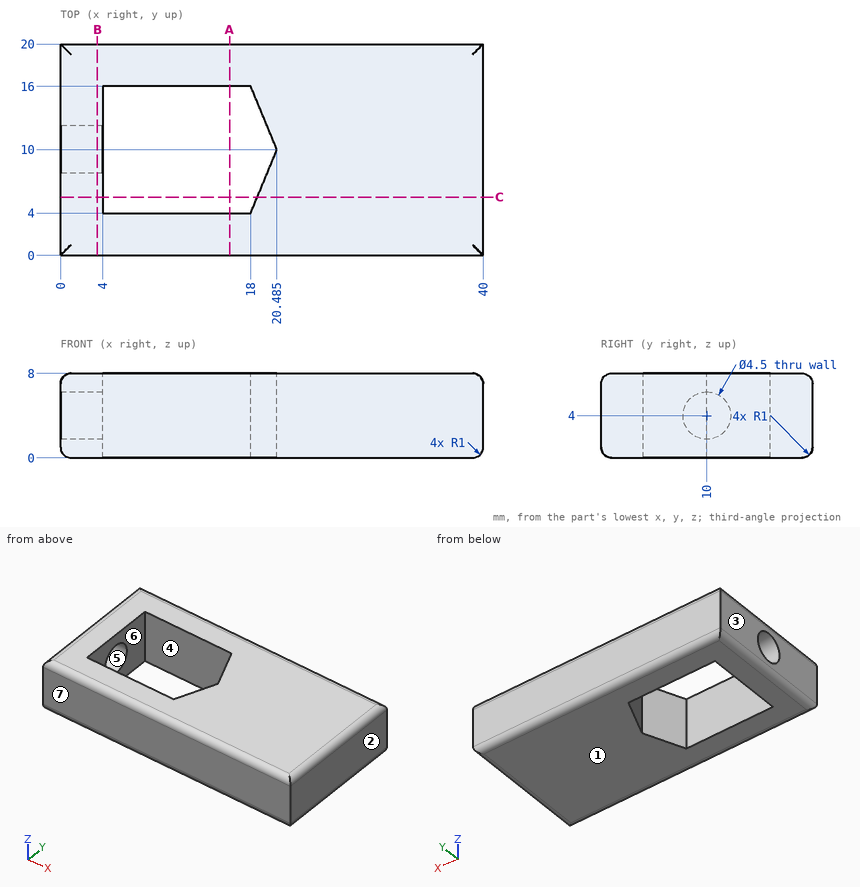
Study the drawing (mm; zero at the part's minimum x, y, z) and answer. A direction names the side the tool comes from. Coordinates: 2 decimals unless noted, no trailing zeros. Order: outer loops, then holes, each group sorted by start corner. A loop starts at its lowest first (then second) coordinate and runs counter-clockwise, first axis right, second up. Notation, with made-up numbers: M 68.5,66 L 127.5,66 A17 cw 127.5,81 Z; hole C -23,-14.5 d3. An arc over 180 degrees is marked long. Answer as a JSON object with one key per item and string values. Group by question number.
1. Section A-A on x = 16 is taken. Write down the section's boundary in (y, z).
2. Determine the mould class of the marked faces 1, 2, 3 and 4 for opening direction X: released by +X, released by -X, zero draft, split by the parting line, or undercut.
3. Straight lines are drawn through the part: line 1 (Y direction, x = 1.95, z = 4); line 2 (Y direction, x = 6.5, z = 1); line 3 (X direction, y = 4.25, z = 1.5). For each, find the intervals that lie inside material, in ascending order.
4. A flat-ended cylindrical pin translates along its axis: P1, Ø12, axis at x = 20, y = 9, coming from the +Z side. Find the tip coordinate at first contact, or state that the pin passes through.
5. A tool of negligible diameter and unlimited length cuts with its end or side. For the marked faces 5, 6 and 7, from which of +Z, -Z, +X, -X, +Y, -Y can it reach the whole face along a straight path? Write none if from no direction.
6. Section C-C on y = 5.5 is taken. Write down the section's boundary in (x, z), then the cut area to 3 significant figures.
7. Section B-B on x = 3.5 is taken. Write down the section's boundary in (y, z), then the cut area to 3 significant figures.
Values follow:
{
 "1": {"outline": "M 0,1 A1 ccw 1,0 L 4,0 L 4,8 L 1,8 A1 ccw 0,7 Z; M 16,0 L 19,0 A1 ccw 20,1 L 20,7 A1 ccw 19,8 L 16,8 Z"},
 "2": {"face 1": "zero draft", "face 2": "released by +X", "face 3": "released by -X", "face 4": "undercut"},
 "3": {"line 1": "0 to 7.75, 12.25 to 20", "line 2": "0 to 4, 16 to 20", "line 3": "0 to 4, 18.1 to 40"},
 "4": {"P1": "z = 8"},
 "5": {"face 5": "-X", "face 6": "+Z, -Z", "face 7": "+Z, -Z, +X, -X, -Y"},
 "6": {"outline": "M 0,1 A1 ccw 1,0 L 4,0 L 4,8 L 1,8 A1 ccw 0,7 Z; M 18.62,0 L 39,0 A1 ccw 40,1 L 40,7 A1 ccw 39,8 L 18.62,8 Z", "area": "202 mm2"},
 "7": {"outline": "M 0,1 A1 ccw 1,0 L 19,0 A1 ccw 20,1 L 20,7 A1 ccw 19,8 L 1,8 A1 ccw 0,7 Z; hole C 10,4 d4.5", "area": "143 mm2"}
}
